Read the model definition and answer for the solid it produces. Units are mm, in the model's axes. Face numbers are marked on the shaded views. Give positions to 0.01 mm unless a question says otherwise; leave off trailing zeros. Order: outer loops, then holes, each group sorted by start corner. A loop starts at its lowest first (then second) coordinate and runs counter-clockwise, first axis right, second up. Notation, with made-up numbers: M 79.25,-33.75 L 138.25,-33.75 A25 cw 138.25,-19.75 Z; hole C 9,76.5 d4. An arc over 180 degrees is marked long. One line per item, written item: value. Start each with the question number.
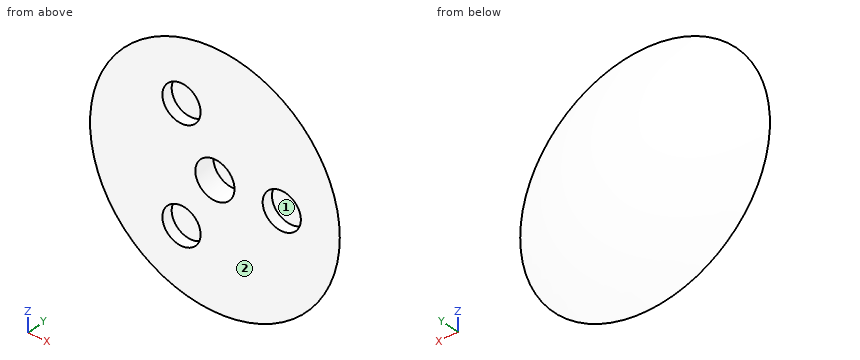
from build123d import *

# Parameters (mm, degrees)
ESQUISSE4_R                  = 10.25
ENL_V_MAT_EXTRU_2_DEPTH      = 11.65
ESQUISSE5_R                  = 10
ENL_V_MAT_EXTRU_3_DEPTH      = 6
R_P_TITION_CIRCULAIRE1_COUNT = 3


with BuildPart() as part:
    # Esquisse1 → Révolution1 (revolve)
    with BuildSketch(Plane.XY):
        with BuildLine():
            Line((0, 15), (0, 0))
            Line((0, 0), (65.383484153, 0))
            ThreePointArc((65.383484153, 0), (33.541019662, 11.201915172), (0, 15))
        make_face()
    revolve(axis=Axis((0, 15, 0), (0, -1, 0)))

    # Esquisse4 → Enlèv. mat.-Extru.2 (cut)
    with BuildSketch(Plane.XZ):
        Circle(ESQUISSE4_R)
    extrude(amount=-ENL_V_MAT_EXTRU_2_DEPTH, mode=Mode.SUBTRACT)

    # Esquisse5 → Enlèv. mat.-Extru.3 (cut)
    with BuildSketch(Plane.XZ):
        with Locations((35, 0)):
            Circle(ESQUISSE5_R)
    enl_v_mat_extru_3 = extrude(amount=-ENL_V_MAT_EXTRU_3_DEPTH, mode=Mode.SUBTRACT)

    # Répétition circulaire1: Enlèv. mat.-Extru.3 ×3 about axis
    r_p_tition_circulaire1_axis = Axis((0, 0, 0), (0, 1, 0))
    for i in range(1, R_P_TITION_CIRCULAIRE1_COUNT):
        add(enl_v_mat_extru_3.rotate(r_p_tition_circulaire1_axis, i * 360 / R_P_TITION_CIRCULAIRE1_COUNT), mode=Mode.SUBTRACT)


solid = part.part
Q1. Find section A-A, the plane z = 0. Give the vertices of the cut face in (x, y).
Q2. Find section D-D, the plane y = 9.25. Give the vertices of the cut face in (x, z).
Q3. Find section B-B, the plane x = 0. Give the vertices of the cut face in (y, z).
Q4. Determine the mould class of the marked faces 1 and 2 for opening direction X: released by +X, released by -X, zero draft, split by the parting line, or undercut.
Q5. Consider probe 1 along X at (y, z) = (1, 2); probe 2 along Z at (x, y) = (-17.5, 2.2); probe 3 along Z at (x, y) = (1, 3). Determine where each line is inside the solid, lowest interval first.
Q6. Find section C-C, the plane y = 2.25. Give the vertices of the cut face in (x, z).
Q7. Each of these flat-tipped pins is pushed along its axis until it touches: pin 1 (16 mm diameter, centred on x = -20, z = 27.5, fed in from -Y); pin 2 (3 mm diameter, centred on x = -12, y = 4, fed in from +Z); pin 3 (1.5 mm diameter, centred on x = -23.5, z = -33.5, fed in from +Y); pin 4 (16 mm diameter, centred on x = -17.5, z = -30.31, fed in from -Y). Where does it stop, or does it pass through?
Evaluation:
1. outline: M -65.38,0 L -10.25,0 L -10.25,11.65 L 10.25,11.65 L 10.25,0 L 25,0 L 25,6 L 45,6 L 45,0 L 65.38,0 A150 ccw Z
2. outline: C 0,0 d82.27; hole C 0,0 d20.5
3. outline: M 0,-65.38 A150 ccw 0,65.38 L 0,10.25 L 11.65,10.25 L 11.65,-10.25 L 0,-10.25 Z
4. face 1: undercut
4. face 2: zero draft
5. probe 1: -63.25 to -10.05, 10.05 to 25.2, 44.8 to 63.25
5. probe 2: -58.05 to -40.31, -20.31 to 20.31, 40.31 to 58.05
5. probe 3: -58.78 to -10.2, 10.2 to 58.78
6. outline: C 0,0 d121.04; hole C -17.5,-30.31 d20; hole C -17.5,30.31 d20; hole C 0,0 d20.5; hole C 35,0 d20
7. pin 1: y = 0
7. pin 2: z = 58.75
7. pin 3: y = 9.52
7. pin 4: y = 6
